Part model, mm, in its own coordinate system. Face numbers are marked on the shaded views. Coordinates: 2 decimals unless noted, no trailing zeros. Loops run counter-clockwise (first coordinate to the right, second up) from the corner with the lowest first, then second, coordinate; pieces in that order, holes last.
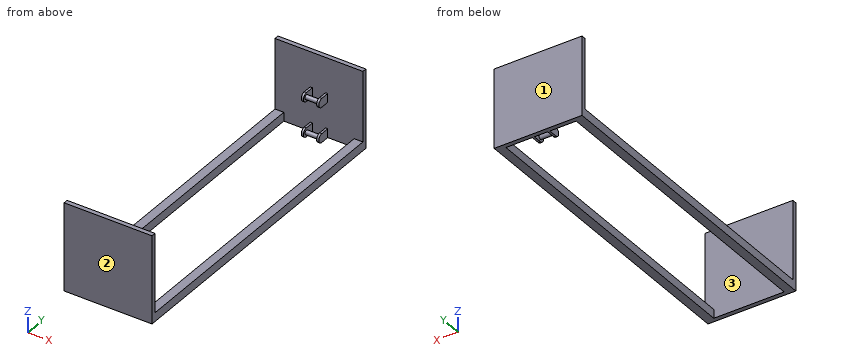
```python
from build123d import *

# Parameters (mm, degrees)
SKETCH2_W           = 200
SKETCH2_H           = 200
BOSS_EXTRUDE1_DEPTH = 10
SKETCH3_W           = 20
SKETCH3_H           = 20
BOSS_EXTRUDE2_DEPTH = 700
SKETCH4_W           = 200
SKETCH4_H           = 180
BOSS_EXTRUDE3_DEPTH = 10
SKETCH5_W           = 40
SKETCH5_H           = 10
BOSS_EXTRUDE4_DEPTH = 20
SKETCH7_R           = 10
BOSS_EXTRUDE7_DEPTH = 40
SKETCH10_W          = 30
SKETCH10_H          = 40.281697436
CUT_EXTRUDE2_DEPTH  = 754.923072999
SKETCH11_R          = 5
BOSS_EXTRUDE9_DEPTH = 40
LPATTERN1_COUNT     = 2
LPATTERN1_PITCH     = 80


with BuildPart() as part:
    # Sketch2 → Boss-Extrude1 (new body)
    with BuildSketch(Plane(origin=(0, 0, 0), x_dir=(1, 0, 0), z_dir=(0, 1, 0))):
        with Locations((100, 100)):
            Rectangle(SKETCH2_W, SKETCH2_H)
    extrude(amount=BOSS_EXTRUDE1_DEPTH)

    # Sketch3 → Boss-Extrude2 (add)
    with BuildSketch(Plane(origin=(0, 10, 0), x_dir=(1, 0, 0), z_dir=(0, 1, 0))):
        with Locations((190, 190)):
            Rectangle(SKETCH3_W, SKETCH3_H)
        with Locations((10, 190)):
            Rectangle(SKETCH3_W, SKETCH3_H)
    extrude(amount=BOSS_EXTRUDE2_DEPTH)

    # Sketch4 → Boss-Extrude3 (add)
    with BuildSketch(Plane(origin=(0, 710, 0), x_dir=(1, 0, 0), z_dir=(0, 1, 0))):
        with Locations((100, 110)):
            Rectangle(SKETCH4_W, SKETCH4_H)
    extrude(amount=BOSS_EXTRUDE3_DEPTH)

    # Sketch5 → Boss-Extrude4 (add)
    with BuildSketch(Plane.XZ.offset(-710)):
        with Locations((100, -105)):
            Rectangle(SKETCH5_W, SKETCH5_H)
        with Locations((100, -115)):
            Rectangle(SKETCH5_W, SKETCH5_H)
    boss_extrude4 = extrude(amount=BOSS_EXTRUDE4_DEPTH)

    # Sketch7 → Boss-Extrude7 (add)
    with BuildSketch(Plane(origin=(120, 0, 0), x_dir=(0, 0, -1), z_dir=(1, 0, 0))):
        with Locations((110, 690)):
            Circle(SKETCH7_R)
    boss_extrude7 = extrude(amount=-BOSS_EXTRUDE7_DEPTH)

    # Sketch10 → Cut-Extrude2 (cut, through all)
    with BuildSketch(Plane.XY.offset(-100)):
        with Locations((100, 689.859151282)):
            Rectangle(SKETCH10_W, SKETCH10_H)
    cut_extrude2 = extrude(amount=-CUT_EXTRUDE2_DEPTH, mode=Mode.SUBTRACT)

    # Sketch11 → Boss-Extrude9 (add)
    with BuildSketch(Plane(origin=(120, 0, 0), x_dir=(0, 0, -1), z_dir=(1, 0, 0))):
        with Locations((110, 690)):
            Circle(SKETCH11_R)
    boss_extrude9 = extrude(amount=-BOSS_EXTRUDE9_DEPTH)

    # LPattern1: Boss-Extrude4, Boss-Extrude7, Cut-Extrude2, Boss-Extrude9 ×2
    with Locations(*[(0, 0, -i * LPATTERN1_PITCH) for i in range(1, LPATTERN1_COUNT)]):
        add(boss_extrude4)
        add(boss_extrude7)
        add(cut_extrude2, mode=Mode.SUBTRACT)
        add(boss_extrude9)


solid = part.part
```
Q1. Probe line 1 (Y direction, x = 138.5, z = -152.5); line 2 (X direction, y = 133.5, z = -185); line 3 (Z direction, x = 187, y = 476). List the from-to ranges inside material, lowest first.
Q2. Saw through at B-B (z = -171). List the corners of the cut face in (x, y).
Q3. Saw through at A-A (x = 161). List the corners of the cut face in (y, z).
Q4. Drop flat-ended pins along their axis: P1, Ø4, axis at x = 83.5, y = 703.5, coming from the +Z side; P2, Ø6, axis at y = 701, z = -108, coming from the -X side; P3, Ø10, axis at x = 7.5, y = 201.5, coming from the +Z side. Give the stop position or say it passes through.
Q5. Mould opens along Y. For the marked faces 1, 2 and 3 say: released by +Y, released by -Y, zero draft, split by the parting line, or undercut.
Q6. Saw through at C-C (x = 98). List the corners of the cut face in (y, z).
Checked values:
1. line 1: y = 0 to 10, 710 to 720
1. line 2: x = 0 to 20, 180 to 200
1. line 3: z = -200 to -180
2. outline: (0, 0) - (200, 0) - (200, 10) - (0, 10) - close; (0, 710) - (200, 710) - (200, 720) - (0, 720) - close
3. outline: (0, -200) - (10, -200) - (10, 0) - (0, 0) - close; (710, -200) - (720, -200) - (720, -20) - (710, -20) - close
4. P1: stops at z = -100
4. P2: stops at x = 80
4. P3: stops at z = -180
5. face 1: released by +Y
5. face 2: released by -Y
5. face 3: undercut
6. outline: (0, -200) - (10, -200) - (10, 0) - (0, 0) - close; circle Ø10 at (690, -190); circle Ø10 at (690, -110); (710, -200) - (720, -200) - (720, -20) - (710, -20) - close
